```python
from build123d import *

# Parameters (mm, degrees)
F0_R     = 3.175
F1_DEPTH = 3.048


with BuildPart() as f1:
    # F0 (on Front) → F1 (new body)
    with BuildSketch(Plane.XZ):
        with BuildLine():
            ThreePointArc((0.9317650018, -83.8459721666), (6.9288640955, -80.8176490707), (9.3440798747, -74.5484648293))
            ThreePointArc((9.3440798747, -74.5484648293), (-0.4451715738, -65.2149954328), (-9.3016620588, -75.4377969659))
            ThreePointArc((-9.3016620588, -75.4377969659), (-6.4238009338, -81.334230097), (-0.3786177199, -83.884870847))
            Line((-0.3786177199, -83.884870847), (0.9317650018, -83.8459721666))
        make_face()
        with Locations((0, -74.5484648293)):
            Circle(F0_R, mode=Mode.SUBTRACT)
        with BuildLine():
            ThreePointArc((-9.3016620588, -75.4377969659), (-0.4451715738, -65.2149954328), (9.3440798747, -74.5484648293))
            ThreePointArc((9.3440798747, -74.5484648293), (6.9288640955, -80.8176490707), (0.9317650018, -83.8459721666))
            Line((0.9317650018, -83.8459721666), (44.45, -82.554134379))
            ThreePointArc((44.45, -82.554134379), (36.5137551878, -74.4754800988), (44.7322639179, -66.6841547333))
            Line((44.7322639179, -66.6841547333), (18.7473772034, -65.7595263374))
            ThreePointArc((18.7473772034, -65.7595263374), (13.0448117515, -63.0471447529), (11.1183414278, -57.0334122443))
            Line((11.1183414278, -57.0334122443), (15.1635767889, -16.051013392))
            ThreePointArc((15.1635767889, -16.051013392), (0.0730961046, -26.9234462481), (-14.9840440257, -16.004887067))
            Line((-14.9840440257, -16.004887067), (-9.3016620588, -75.4377969659))
        make_face()
        with BuildLine():
            ThreePointArc((-0.3786177199, -83.884870847), (0.2772566603, -83.8884304315), (0.9317650018, -83.8459721666))
            Line((0.9317650018, -83.8459721666), (-0.3786177199, -83.884870847))
        make_face()
        with BuildLine():
            Line((-15.6499966361, -9.0395859455), (-14.9840440257, -16.004887067))
            ThreePointArc((-14.9840440257, -16.004887067), (0.0730961046, -26.9234462481), (15.1635767889, -16.051013392))
            Line((15.1635767889, -16.051013392), (15.8508702184, -9.0880233702))
            ThreePointArc((15.8508702184, -9.0880233702), (0.1217952948, 4.8265164035), (-15.6499966361, -9.0395859455))
        make_face()
        with Locations((0.0973850711, -11.0484648293)):
            Circle(F0_R, mode=Mode.SUBTRACT)
        with BuildLine():
            ThreePointArc((-15.6499966361, -9.0395859455), (-15.7055497457, -12.5593838131), (-14.9840440257, -16.004887067))
            Line((-14.9840440257, -16.004887067), (-15.6499966361, -9.0395859455))
        make_face()
        with BuildLine():
            ThreePointArc((44.7322639179, -66.6841547333), (36.5137551878, -74.4754800988), (44.45, -82.554134379))
            ThreePointArc((44.45, -82.554134379), (50.0626600757, -80.2292944547), (52.3875, -74.616634379))
            ThreePointArc((52.3875, -74.616634379), (50.1615836726, -69.1046730039), (44.7322639179, -66.6841547333))
        make_face()
        with Locations((44.45, -74.616634379)):
            Circle(F0_R, mode=Mode.SUBTRACT)
        with BuildLine():
            Line((-9.2905856273, 40.8111409425), (-15.6499966361, -9.0395859455))
            ThreePointArc((-15.6499966361, -9.0395859455), (0.1217952948, 4.8265164035), (15.8508702184, -9.0880233702))
            Line((15.8508702184, -9.0880233702), (9.6411718832, 40.8111409425))
            ThreePointArc((9.6411718832, 40.8111409425), (9.6855013313, 40.2821620908), (9.7002931279, 39.7515351707))
            ThreePointArc((9.7002931279, 39.7515351707), (-0.3553337921, 30.2413269673), (-9.2905856273, 40.8111409425))
        make_face()
        with Locations((-3.1145731919, 25.4767351707)):
            Circle(F0_R, mode=Mode.SUBTRACT)
        with BuildLine():
            Line((15.8508702184, -9.0880233702), (15.1635767889, -16.051013392))
            ThreePointArc((15.1635767889, -16.051013392), (15.7688785947, -13.5822200937), (15.9723850711, -11.0484648293))
            ThreePointArc((15.9723850711, -11.0484648293), (15.9419772355, -10.0663629285), (15.8508702184, -9.0880233702))
        make_face()
        with BuildLine():
            ThreePointArc((9.6411718832, 40.8111409425), (0.1752931279, 49.2765351707), (-9.2905856273, 40.8111409425))
            ThreePointArc((-9.2905856273, 40.8111409425), (-0.3553337921, 30.2413269673), (9.7002931279, 39.7515351707))
            ThreePointArc((9.7002931279, 39.7515351707), (9.6855013313, 40.2821620908), (9.6411718832, 40.8111409425))
        make_face()
        with Locations((0.1752931279, 39.7515351707)):
            Circle(F0_R, mode=Mode.SUBTRACT)
    extrude(amount=-F1_DEPTH)


solid = f1.part
```
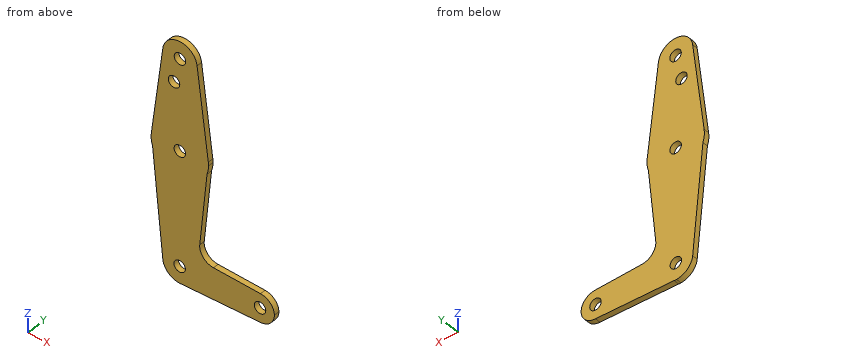
The listing builds one solid part. Answer for the finished solid, in the listing's coordinates (mm). Round coordinates to 2 decimals unless told otherwise and drop trailing zeros. Order: outer loops, then holes, each group sorted by start corner. A loop starts at its lowest first (then second) coordinate and runs counter-clockwise, first axis right, second up. Notation, with made-up numbers: (-34.75, 54) -> (-20.75, 54) arc R18 cw to (-20.75, 70) -> close; hole circle Ø10 at (87.5, 83.25). An arc over 180 degrees is marked (long way). Answer as CSV lines item,"result".
Q1. A cutting plane is placed at A-A on y = 1.2. Give the number of separate pieces and of enclosed holes in the cut face, plus the area to 3 significant figures.
Computed values:
separate pieces,"1"
enclosed holes,"5"
area,"3,730 mm^2"
Q2. Given pin 1 (1.5 mm diameter, centred on x = 4, y = 2.5, fed in from +Z), flat-ended and moving along its own axis, determine where the tip first touches the part or whether it passes through.
Computed values:
pin 1,"stops at z = 48.77"
Q3. A cutting plane is placed at D-D on x = 21. Determine the outline of the cut face in (y, z), plus the area to 3 significant figures.
Computed values:
outline,"(0, -83.25) -> (3.05, -83.25) -> (3.05, -65.84) -> (0, -65.84) -> close"
area,"53.1 mm^2"
Q4. A cutting plane is placed at C-C on z = 15. Determine the outline of the cut face in (x, y).
Computed values:
outline,"(-12.58, 0) -> (12.85, 0) -> (12.85, 3.05) -> (-12.58, 3.05) -> close"
Q5. Consider line 1 (Z direction, x = -2, y = 0.9); line 2 (X direction, y = 1.55, z = -76); line 3 (Z direction, x = -5.5, y = 2.75). Determine where each line is inside the solid, lowest interval first. Write a range as from..to.
Computed values:
line 1,"z = -83.68..-77.01, -72.08..-13.43, -8.66..22.5, 28.45..37.44, 42.06..49.02"
line 2,"x = -9.23..-2.82, 2.82..41.59, 47.31..52.27"
line 3,"z = -82.1..23.38, 27.57..47.4"
Q6. A cutting plane is placed at B-B on x = 43. Determine the outline of the cut face in (y, z), plus the area to 3 significant figures.
Computed values:
outline,"(0, -82.6) -> (3.05, -82.6) -> (3.05, -77.44) -> (0, -77.44) -> close; (0, -71.79) -> (3.05, -71.79) -> (3.05, -66.62) -> (0, -66.62) -> close"
area,"31.5 mm^2"
